Geometry: see drawing. Coordinates: mm, zero at the bounding-box minimum. A direction names the side the tool comes from. Coordinates: 2 decimals unless noted, no trailing zeros. Order: outer loops, then holes, each group sorted by start corner. A loop starts at its lowest first (then second) coordinate and runs counter-clockwise, first axis right, second up.
Item 1: Section B-B on x = 92. Return the cut outline in (y, z).
Item 2: Ray query, line 1 (X direction, y = 57.5, z = 36.5); line 2 (Y direction, x = 75.5, z = 38); line 3 (Z direction, x = 110, y = 39). Return the intervals inside material, ascending.
Item 3: Contact query for flat-ended pins moving along their axis: P1, Ø5, axis at x = 81.5, y = 43.5, coming from the +Z side; P2, Ø6, axis at y = 13.5, z = 61.5, coming from the -X side; P3, Ø8, axis at x = 139.5, y = 64.5, coming from the +Z side; P4, Ø8, axis at x = 100.5, z = 24.5, coming from the +Y side. Output: stop coordinate, or through.
Item 4: Reachability of the marked faces 4 and 5 from +Z, -Z, +X, -X, +Y, -Y: full face, straight path, thin tool, end or side. Return the list, or none.
Item 5: Mould query, pull axis X, two halves, no side actions, for the marked faces 1, 2 and 3. Classes: released by +X, released by -X, zero draft, split by the parting line, or undercut.
Item 6: Section A-A on x = 18. Return the cut outline in (y, z).
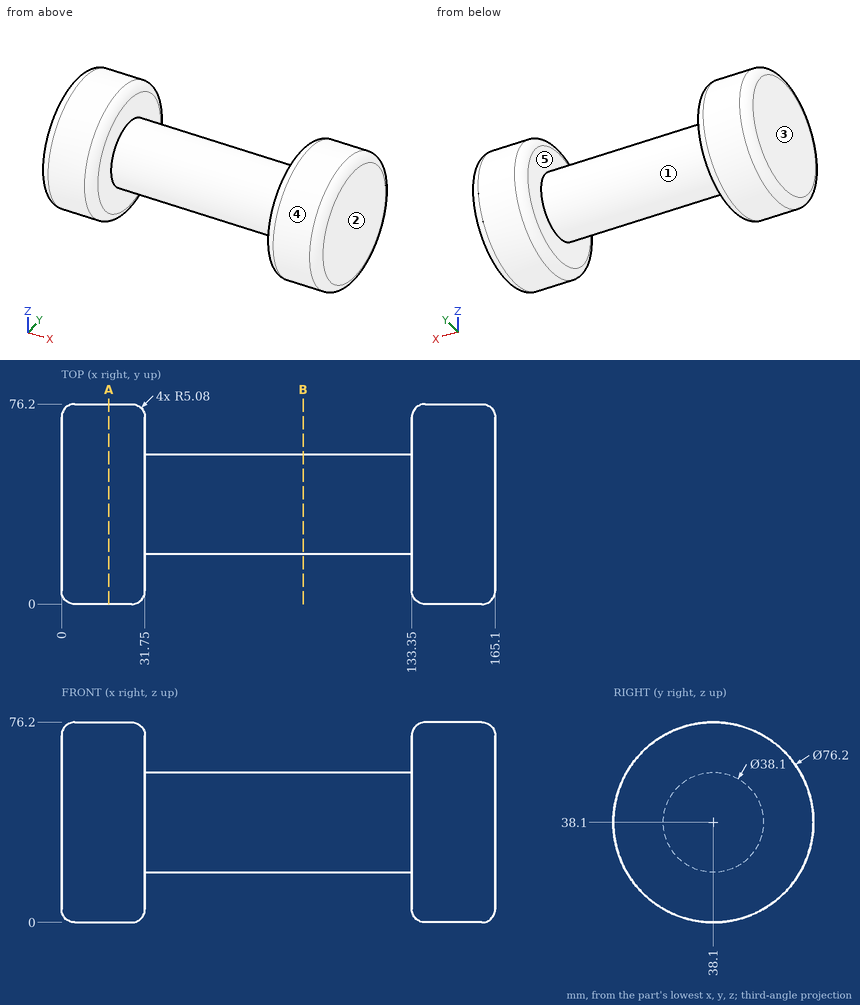
Answer list:
1. outline: circle Ø38.1 at (38.1, 38.1)
2. line 1: x = 0 to 31.75, 133.35 to 165.1
2. line 2: y = 19.05 to 57.15
2. line 3: z = 19.07 to 57.13
3. P1: stops at z = 56.93
3. P2: stops at x = 0
3. P3: stops at z = 68.92
3. P4: stops at y = 54.55
4. face 4: +X, -X
4. face 5: none
5. face 1: undercut
5. face 2: released by +X
5. face 3: released by -X
6. outline: circle Ø76.2 at (38.1, 38.1)
